```python
from build123d import *

# Parameters (mm, degrees)
SKETCH1_R                       = 15
BOSS_EXTRUDE2_DEPTH             = 8.255
BOSS_EXTRUDE3_DEPTH             = 8.255
SKETCH5_R                       = 3.249999977
CUT_EXTRUDE3_DEPTH              = 63.5
SKETCH7_W                       = 3.175
SKETCH7_H                       = 25.4
BOSS_EXTRUDE5_DEPTH             = 19.05
CUT_EXTRUDE6_DEPTH              = 149.35
CIRPATTERN2_COUNT               = 2
CIRPATTERN2_ANGLE               = 90
CIRPATTERN3_COUNT               = 2
CIRPATTERN3_ANGLE               = 90
BOSS_EXTRUDE6_DEPTH             = 8.255
BOSS_EXTRUDE7_REACH             = 21.05
BOSS_EXTRUDE7_DIRECTION_2_REACH = 135.35
BOSS_EXTRUDE8_REACH             = 21.05
BOSS_EXTRUDE8_DIRECTION_2_REACH = 135.35
BOSS_EXTRUDE9_REACH             = 133.763
SKETCH19_W                      = 3.81
SKETCH19_H                      = 8.255
BOSS_EXTRUDE10_REACH            = 133.763
SKETCH20_W                      = 3.81
SKETCH20_H                      = 8.255


with BuildPart() as part:
    # Sketch1 → Boss-Extrude2 (new body)
    with BuildSketch(Plane(origin=(0, 0, 0), x_dir=(1, 0, 0), z_dir=(0, 1, 0))):
        Circle(SKETCH1_R)
    extrude(amount=BOSS_EXTRUDE2_DEPTH)

    # Sketch1<6> → Boss-Extrude3 (add)
    with BuildSketch(Plane(origin=(0, 0, 0), x_dir=(1, 0, 0), z_dir=(0, 1, 0))):
        with BuildLine():
            Line((-1.5875, 130.175), (-1.5875, 14.915758236))
            ThreePointArc((-1.5875, 14.915758236), (0, 15), (1.5875, 14.915758236))
            Line((1.5875, 14.915758236), (1.5875, 130.175))
            Line((1.5875, 130.175), (-1.5875, 130.175))
        make_face()
        with BuildLine():
            ThreePointArc((-14.915758236, -1.5875), (-15, 0), (-14.915758236, 1.5875))
            Line((-14.915758236, 1.5875), (-130.175, 1.5875))
            Line((-130.175, 1.5875), (-130.175, -1.5875))
            Line((-130.175, -1.5875), (-14.915758236, -1.5875))
        make_face()
    extrude(amount=BOSS_EXTRUDE3_DEPTH)

    # Sketch5 → Cut-Extrude3 (cut)
    with BuildSketch(Plane(origin=(0, 8.255, 0), x_dir=(1, 0, 0), z_dir=(0, 1, 0))):
        Circle(SKETCH5_R)
        with BuildLine():
            Line((-5.908712478, 5.423058993), (-7.721732332, 7.873214705))
            ThreePointArc((-7.721732332, 7.873214705), (-7.403164404, 10.004802487), (-5.271576621, 9.686234559))
            Line((-5.271576621, 9.686234559), (-3.458556767, 7.236078848))
            ThreePointArc((-3.458556767, 7.236078848), (-3.777124696, 5.104491065), (-5.908712478, 5.423058993))
        make_face()
        with BuildLine():
            Line((3.458556767, -7.236078848), (5.271576621, -9.686234559))
            ThreePointArc((5.271576621, -9.686234559), (7.403164404, -10.004802487), (7.721732332, -7.873214705))
            Line((7.721732332, -7.873214705), (5.908712478, -5.423058993))
            ThreePointArc((5.908712478, -5.423058993), (3.777124696, -5.104491065), (3.458556767, -7.236078848))
        make_face()
    extrude(amount=-CUT_EXTRUDE3_DEPTH, mode=Mode.SUBTRACT)

    # Sketch7 → Boss-Extrude5 (add, symmetric)
    with BuildSketch(Plane(origin=(0, 0, 0), x_dir=(0, 0, -1), z_dir=(1, 0, 0))):
        with Locations((131.7625, 12.7)):
            Rectangle(SKETCH7_W, SKETCH7_H)
    boss_extrude5 = extrude(amount=BOSS_EXTRUDE5_DEPTH, both=True)

    # Sketch12 → Cut-Extrude6 (cut, through all)
    with BuildSketch(Plane(origin=(0, 0, -133.35), x_dir=(-1, 0, 0), z_dir=(0, 0, -1))):
        with BuildLine():
            Line((-6.35, 10.541), (-12.7, 10.541))
            ThreePointArc((-12.7, 10.541), (-14.859, 12.7), (-12.7, 14.859))
            Line((-12.7, 14.859), (-6.35, 14.859))
            ThreePointArc((-6.35, 14.859), (-4.191, 12.7), (-6.35, 10.541))
        make_face()
        with BuildLine():
            Line((6.35, 14.859), (12.7, 14.859))
            ThreePointArc((12.7, 14.859), (14.859, 12.7), (12.7, 10.541))
            Line((12.7, 10.541), (6.35, 10.541))
            ThreePointArc((6.35, 10.541), (4.191, 12.7), (6.35, 14.859))
        make_face()
    cut_extrude6 = extrude(amount=-CUT_EXTRUDE6_DEPTH, mode=Mode.SUBTRACT)

    # CirPattern2: Boss-Extrude5 ×2 about axis
    cirpattern2_axis = Axis((0, 0, 0), (0, 1, 0))
    for i in range(1, CIRPATTERN2_COUNT):
        add(boss_extrude5.rotate(cirpattern2_axis, i * CIRPATTERN2_ANGLE / (CIRPATTERN2_COUNT - 1)))

    # CirPattern3: Cut-Extrude6 ×2 about axis
    cirpattern3_axis = Axis((0, 0, 0), (0, 1, 0))
    for i in range(1, CIRPATTERN3_COUNT):
        add(cut_extrude6.rotate(cirpattern3_axis, i * CIRPATTERN3_ANGLE / (CIRPATTERN3_COUNT - 1)), mode=Mode.SUBTRACT)

    # Sketch13 → Boss-Extrude6 (add)
    with BuildSketch(Plane.XZ):
        Polygon((-96.628948776, -1.5875), (-1.5875, -96.628948776), (-1.5875, -100.221051224), (-100.221051224, -1.5875), align=None)
        Polygon((-19.05, -130.175), (-1.5875, -115.831500599), (-1.5875, -119.118499401), (-15.048241783, -130.175), align=None)
        Polygon((19.05, -130.175), (1.5875, -115.831500599), (1.5875, -119.118499401), (15.048241783, -130.175), align=None)
        Polygon((-119.118499401, 1.5875), (-130.175, 15.048241783), (-130.175, 19.05), (-115.831500599, 1.5875), align=None)
        Polygon((-119.118499401, -1.5875), (-130.175, -15.048241783), (-130.175, -19.05), (-115.831500599, -1.5875), align=None)
    extrude(amount=-BOSS_EXTRUDE6_DEPTH)

    # Boss-Extrude7: up to this face of the body (flat: up to its plane)
    boss_extrude7_end = Plane(part.part.faces().sort_by_distance((-124.646749701, 4.1275, 1.5875))[0])
    # Sketch14 → Boss-Extrude7 (add, up to the picked face)
    with BuildSketch(Plane.XY, mode=Mode.PRIVATE) as boss_extrude7_sk1:
        Polygon((-130.175, 25.4), (-117.475, 8.255), (-130.175, 8.255), align=None)
    boss_extrude7_tool1 = split(extrude(boss_extrude7_sk1.sketch, amount=BOSS_EXTRUDE7_REACH, mode=Mode.PRIVATE), bisect_by=boss_extrude7_end, keep=Keep.BOTH, mode=Mode.PRIVATE)
    add(boss_extrude7_tool1.solids().sort_by_distance((-125.941667, 13.97, 0))[0])

    # Boss-Extrude7 direction 2: up to this face of the body (flat: up to its plane)
    boss_extrude7_direction_2_end = Plane(part.part.faces().sort_by_distance((-124.646749701, 4.1275, -1.5875))[0])
    # Sketch14 → Boss-Extrude7 direction 2 (add, up to the picked face)
    with BuildSketch(Plane.XY, mode=Mode.PRIVATE) as boss_extrude7_direction_2_sk1:
        Polygon((-130.175, 25.4), (-117.475, 8.255), (-130.175, 8.255), align=None)
    boss_extrude7_direction_2_tool1 = split(extrude(boss_extrude7_direction_2_sk1.sketch, amount=-BOSS_EXTRUDE7_DIRECTION_2_REACH, mode=Mode.PRIVATE), bisect_by=boss_extrude7_direction_2_end, keep=Keep.BOTH, mode=Mode.PRIVATE)
    add(boss_extrude7_direction_2_tool1.solids().sort_by_distance((-125.941667, 13.97, 0))[0])

    # Boss-Extrude8: up to this face of the body (flat: up to its plane)
    boss_extrude8_end = Plane(part.part.faces().sort_by_distance((1.5875, 4.1275, -65.373629417))[0])
    # Sketch15 → Boss-Extrude8 (add, up to the picked face)
    with BuildSketch(Plane(origin=(0, 0, 0), x_dir=(0, 0, -1), z_dir=(1, 0, 0)), mode=Mode.PRIVATE) as boss_extrude8_sk1:
        Polygon((130.175, 25.4), (115.831500599, 8.255), (130.175, 8.255), align=None)
    boss_extrude8_tool1 = split(extrude(boss_extrude8_sk1.sketch, amount=BOSS_EXTRUDE8_REACH, mode=Mode.PRIVATE), bisect_by=boss_extrude8_end, keep=Keep.BOTH, mode=Mode.PRIVATE)
    add(boss_extrude8_tool1.solids().sort_by_distance((0, 13.97, -125.393834))[0])

    # Boss-Extrude8 direction 2: up to this face of the body (flat: up to its plane)
    boss_extrude8_direction_2_end = Plane(part.part.faces().sort_by_distance((-1.5875, 4.1275, -108.026275912))[0])
    # Sketch15 → Boss-Extrude8 direction 2 (add, up to the picked face)
    with BuildSketch(Plane(origin=(0, 0, 0), x_dir=(0, 0, -1), z_dir=(1, 0, 0)), mode=Mode.PRIVATE) as boss_extrude8_direction_2_sk1:
        Polygon((130.175, 25.4), (115.831500599, 8.255), (130.175, 8.255), align=None)
    boss_extrude8_direction_2_tool1 = split(extrude(boss_extrude8_direction_2_sk1.sketch, amount=-BOSS_EXTRUDE8_DIRECTION_2_REACH, mode=Mode.PRIVATE), bisect_by=boss_extrude8_direction_2_end, keep=Keep.BOTH, mode=Mode.PRIVATE)
    add(boss_extrude8_direction_2_tool1.solids().sort_by_distance((0, 13.97, -125.393834))[0])

    # Sketch19 → Boss-Extrude9 (add, up to next)
    with BuildSketch(Plane.ZY.offset(1.5875), mode=Mode.PRIVATE) as boss_extrude9_sk1:
        with Locations((-55.809758236, 4.1275)):
            Rectangle(SKETCH19_W, SKETCH19_H)
    boss_extrude9_tool1 = extrude(boss_extrude9_sk1.sketch, amount=BOSS_EXTRUDE9_REACH, mode=Mode.PRIVATE) - part.part
    add(boss_extrude9_tool1.solids().sort_by_distance((-1.5875, 4.1275, -55.809758))[0])

    # Sketch20 → Boss-Extrude10 (add, up to next)
    with BuildSketch(Plane(origin=(0, 0, -1.5875), x_dir=(-1, 0, 0), z_dir=(0, 0, -1)), mode=Mode.PRIVATE) as boss_extrude10_sk1:
        with Locations((55.809758236, 4.1275)):
            Rectangle(SKETCH20_W, SKETCH20_H)
    boss_extrude10_tool1 = extrude(boss_extrude10_sk1.sketch, amount=BOSS_EXTRUDE10_REACH, mode=Mode.PRIVATE) - part.part
    add(boss_extrude10_tool1.solids().sort_by_distance((-55.809758, 4.1275, -1.5875))[0])


solid = part.part
```
Geometry check sheet. Reference: the model listing, model coordinates, mm. A direction names the side the tool comes from. Round coordinates to 2 decimals unless told otherwise and drop trailing zeros. Loops run counter-clockwise (first coordinate to the right, second up) from the corner with the lowest first, then second, coordinate; pieces in that order, holes last. Notation, with made-up numbers: (72, 20) - (100, 20) arc R20 cw to (100, 43) - close; hole circle Ø3 at (12.5, 49.25). An arc over 180 degrees is marked (long way). Write item = value, one per line. Start each with the question number.
1. Depth check by flat-ended pin: pin 1 (1.5 mm diameter, centred on x = -20, y = 5.5, fed in from -Z); pin 2 (6.5 mm diameter, centred on x = -86.5, y = 4, fed in from -Z); pin 3 (4 mm diameter, centred on y = 2.5, z = -108.5, fed in from -X); pin 4 (4 mm diameter, centred on y = 11, z = -63, fed in from +X). Enter the tip coordinate at first touch or a pass-through.
2. Thickness scan on line 1 (X direction, y = 2, z = 0); line 2 (Z direction, x = -118, y = 3.25). Record the ranges inside material, lowest first.
3. Mould release check, pull along Z, two halves, no side actions. Record for faces 5 (the face through (0.022, 16.948, -123.104)), 6 (the face through (-124.569, 4.07, 8.224)), 7 (the face through (-123.914, 16.948, 0.022)): released by +Z, released by -Z, zero draft, split by the parting line, or undercut.
4. Section check A-A on z = -26.5. Enter the section's corners in (x, y) (1 decimal).
5. Section check C-C on z = -62. Enter the section's corners in (x, y) (1 decimal), then the cut area to 3 significant figures.
6. Set-up check for faces 1 (the face through (-123.104, 4.07, 10.441)), 2 (the face through (10.441, 4.07, -123.104)), 3 (the face through (-49.175, 4.07, -49.041)), 4 (the face through (-1.588, 4, -108)): record each of +Z, -Z, +X, -X, +Y, -Y from which the full face is reachable in a straight line by a thin tool's end or side.
Working result:
q1.pin_1 = -82.56
q1.pin_2 = -18.56
q1.pin_3 = -1.59
q1.pin_4 = through
q2.line_1 = -133.35 to -3.25, 3.25 to 15
q2.line_2 = -4.23 to 4.23
q3.face_5 = released by +Z
q3.face_6 = undercut
q3.face_7 = zero draft
q4.outline = (-75.3, 0) - (-71.7, 0) - (-71.7, 8.3) - (-75.3, 8.3) - close; (-57.7, 0) - (-53.9, 0) - (-53.9, 8.3) - (-57.7, 8.3) - close; (-1.6, 0) - (1.6, 0) - (1.6, 8.3) - (-1.6, 8.3) - close
q5.outline = (-39.8, 0) - (-36.2, 0) - (-36.2, 8.3) - (-39.8, 8.3) - close; (-1.6, 0) - (1.6, 0) - (1.6, 8.3) - (-1.6, 8.3) - close
q5.area = 55.9 mm^2
q6.face_1 = +Z, +Y, -Y
q6.face_2 = +X, +Y, -Y
q6.face_3 = +Y, -Y
q6.face_4 = -X, +Y, -Y
